Here's how the part is built. I have some questions about the finished solid (model axes, mm). A direction names the side the tool comes from. Give positions to 0.01 mm unless a question says otherwise; leave off trailing zeros. Loops run counter-clockwise (first coordinate to the right, second up) from the corner with the lowest first, then second, coordinate; pieces in that order, holes last. Notation, with made-up numbers: M 62.5,-26 L 72.5,-26 A21 cw 72.5,-17 Z; hole C -20.5,58.5 d8. An arc over 180 degrees is marked long. Write item = value, one per line. Start each with the question number.
```python
from build123d import *

# Parameters (mm, degrees)
F0_R     = 12.15
F1_DEPTH = 4.45


with BuildPart() as f1:
    # F0 (on Top) → F1 (new body)
    with BuildSketch(Plane.XY):
        Polygon((50, -33.5685), (50, -16.64242), (50, 16.64242), (50, 33.5685), (50, 34.008425), (50, 38.0185), (33.6925, 38.0185), (33.6925, 34.008425), (-33.6925, 33.5685), (-33.6925, 38.0185), (-50, 38.0185), (-50, 33.5685), (-50, 16.64242), (-50, -16.64242), (-50, -33.5685), (-50, -38.0185), (-50, -42.4685), (-33.6925, -42.4685), (-33.6925, -38.0185), (33.6925, -38.0185), (33.6925, -42.4685), (50, -42.4685), (50, -38.0185), align=None)
        with Locations((0, -14.429661)):
            Circle(F0_R, mode=Mode.SUBTRACT)
        with Locations((-21.987291, 0)):
            Circle(F0_R, mode=Mode.SUBTRACT)
        with Locations((21.987292, 0)):
            Circle(F0_R, mode=Mode.SUBTRACT)
        with Locations((0, 14.429661)):
            Circle(F0_R, mode=Mode.SUBTRACT)
    extrude(amount=F1_DEPTH)


solid = f1.part
```
Q1. On a 3-axis mill with a long thin cutter (end or side, diameter ignored), from which of +Z, -Z, +X, -X, +Y, -Y can I reach the whole of each face in a straight line? I mean faces 1 (the flat face through (33.692, 36, 2)), 2 (the flat face through (-33.692, -40, 2)), 3 (the flat face through (-50, -2, 2)). Say none if no direction works.
Q2. If we section it at B-B, the plane x = 17.5: List the corners of the cut face in (y, z) for me.
Q3. If we section it at C-C, the plane x = 6: List the corners of the cut face in (y, z) for me.
Q4. If I drill on line 1 along X through (y, z) = (-3.5, 3.6); line 2 along Y through (x, z) = (4.5, 1.15); line 3 along X through (y, z) = (-4.5, 3.8), over which ranges is the centre line in solid material (lowest first)?
Q5. If we section it at A-A, the plane y = 0: List the corners of the cut face in (x, z) for me, then the cut area to 3 significant figures.
Q6. We'd pull the mould along Y, two halves only. Please class faces 4 (the flat face through (-42, -42.468, 2)), 5 (the flat face through (33.692, -40, 2)), 6 (the cylindrical face through (-10.4, 3.65, 2.19)): pulls with the +Y half, pulls with the -Y half, needs draft (parallel to the pull), parting line crosses it, or undercut.
Q7. If we section it at D-D, the plane z = 2.4: List the corners of the cut face in (x, y) for me.
Q8. Will this pin go through, and if not, where does the flat tip stop? pin 1 (2 mm diameter, centred on x = 14.5, z = 1.5, fed in from -Y).
Resolved:
q1.face_1 = +Z, -Z, +Y
q1.face_2 = +Z, -Z, -Y
q1.face_3 = +Z, -Z, -X, +Y, -Y
q2.outline = M -38.02,0 L -11.29,0 L -11.29,4.45 L -38.02,4.45 Z; M 11.29,0 L 33.9,0 L 33.9,4.45 L 11.29,4.45 Z
q3.outline = M -38.02,0 L -24.99,0 L -24.99,4.45 L -38.02,4.45 Z; M -3.86,0 L 3.86,0 L 3.86,4.45 L -3.86,4.45 Z; M 24.99,0 L 33.83,0 L 33.83,4.45 L 24.99,4.45 Z
q4.line_1 = -50 to -33.62, -10.35 to -5.31, 5.31 to 10.35, 33.62 to 50
q4.line_2 = -38.02 to -25.72, -3.14 to 3.14, 25.72 to 33.82
q4.line_3 = -50 to -33.27, -10.7 to -7, 7 to 10.7, 33.27 to 50
q5.outline = M -50,0 L -34.14,0 L -34.14,4.45 L -50,4.45 Z; M -9.84,0 L 9.84,0 L 9.84,4.45 L -9.84,4.45 Z; M 34.14,0 L 50,0 L 50,4.45 L 34.14,4.45 Z
q5.area = 229 mm²
q6.face_4 = pulls with the -Y half
q6.face_5 = needs draft
q6.face_6 = undercut
q7.outline = M -50,-42.47 L -33.69,-42.47 L -33.69,-38.02 L 33.69,-38.02 L 33.69,-42.47 L 50,-42.47 L 50,38.02 L 33.69,38.02 L 33.69,34.01 L -33.69,33.57 L -33.69,38.02 L -50,38.02 Z; hole C -21.99,0 d24.3; hole C 0,-14.43 d24.3; hole C 0,14.43 d24.3; hole C 21.99,0 d24.3
q8.pin_1 = -38.02
